Autodesk Inventor part; units mm, degrees
ref_plane "РабПлоскость6" through (0, -10.8, 0) normal (1, 0, 0) x (0, 0, -1)
ref_plane "YZ Plane" through (0, 0, 0) normal (1, 0, 0) x (0, 1, 0)
ref_plane "XZ Plane" through (0, 0, 0) normal (0, 1, 0) x (-1, 0, 0)
sketch "Эскиз1" plane through (0, 0, 0) normal (0, 0, 1) x (1, 0, 0)
  circle A0 centre (0, 0) radius 5.75
  circle A1 centre (0, 0) radius 9.55
  line L0 (9.55, 13.5) -> (-9.55, 13.5)
  line L1 (-9.55, 13.5) -> (-9.55, 0)
  line L2 (-9.55, 0) -> (9.55, 0)
  line L3 (9.55, 0) -> (9.55, 13.5)
  line L4 (9.55, 0) -> (-9.55, 0)
  line L5 (-9.55, 0) -> (-9.55, -10.8)
  line L6 (-9.55, -10.8) -> (9.55, -10.8)
  line L7 (9.55, -10.8) -> (9.55, 0)
  point P0 (9.55, 0)
  point P1 (0, 9.55)
  point P2 (-9.55, 0)
  point P3 (9.55, 0)
  point P4 (-9.55, 0)
  dimension "d0" = 11.5
  dimension "d1" = 19.1
  dimension "d64" = 10.8
  dimension "d85" = 13.5
extrude "Выдавливание1" add sketch "Эскиз1" along normal blind 8 contours L2 A1 A0 | A0 L2 A1 | L7 L6 L5 A1 | A1 L1 L0 L3
sketch "Эскиз15" plane through (0, 0, 8) normal (0, 0, 1) x (1, 0, 0)
  circle A0 centre (0, 0) radius 5.75
  circle A1 centre (0, 0) radius 7.55
  dimension "d67" = 15.1
extrude "Выдавливание9" cut sketch "Эскиз15" against normal blind 4
ref_plane "РабПлоскость6" through (0, -10.8, 0) normal (1, 0, 0) x (0, 0, -1)
sketch "Эскиз16" plane through (-9.55, -10.8, 0) normal (0, -1, 0) x (1, 0, 0)
  line L0 (0, 8) -> (19.1, 8)
  line L1 (19.1, 8) -> (24.7, 8)
  line L2 (24.7, 8) -> (24.7, 0)
  line L3 (24.7, 0) -> (19.1, 0)
  line L4 (19.1, 0) -> (19.1, 8)
  point P0 (9.55, 0)
  dimension "d70" = 5.6
  dimension "d71" = 8
extrude "Выдавливание10" add sketch "Эскиз16" against normal up to surface (24.3 mm away)
sketch "Эскиз17" plane through (-9.55, 13.5, 0) normal (0, 1, 0) x (1, 0, 0)
  line L0 (24.7, 0) -> (24.7, -8)
  line L1 (24.7, -4) -> (20.15, -4)
  point P0 (9.55, 0)
  dimension "d82" = 4.55
hole "Отверстие4" at (10.6, 13.5, 4) direction (0, -1, 0) diameter 3.2 end through all
fillet "Сопряжение5" radius 5.05 1 edges at (15.15, 1.35, 8)
fillet "Сопряжение5" radius 2.95 1 edges at (15.15, 1.35, 0)
mirror "Зеркальное отражение5" about plane through (0, -10.8, 0) normal (1, 0, 0) of "Сопряжение5", "Отверстие4", "Выдавливание10"
sketch "Эскиз18" plane through (0, 0, 8) normal (0, 0, 1) x (1, 0, 0)
  circle A0 centre (0, 0) radius 7.55
  circle A1 centre (0, 16.1) radius 7.55
  circle A2 centre (0, -16.1) radius 7.55
  dimension "d86" = 16.1
  dimension "d87" = 16.1
extrude "Выдавливание11" cut sketch "Эскиз18" against normal through all contours A1 | A2
ref_plane "РабПлоскость7" through (0, -10.8, 0) normal (1, 0, 0) x (0, 0, -1)
equation "\"d87\" = d86"
properties part number "Крепление дифференциала"
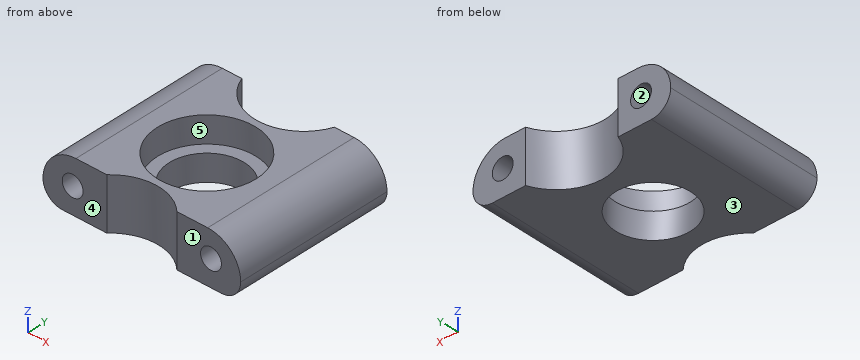
Could you check a few things on this model? Use its own coordinates, in mm. Face numbers are marked on the shaded views. A direction names the side the tool comes from. Give positions to 0.01 mm unless a question says otherwise; leave off trailing zeros. Order: outer loops, then holes, each group sorted by start corner. A loop starts at its lowest first (then second) coordinate and runs counter-clockwise, first axis right, second up.
Q1. Suppose I cut it at B-B, the plane x = 0. Write out the boundary of the cut face in (y, z).
Q2. For the marked faces 4 and 5, which set-ups out of +Z, -Z, +X, -X, +Y, -Y let a thin tool reach every point of the face, with its end or its side?
Q3. Suppose I cut it at A-A, the plane y = 0. Count the separate pieces of the cut face and the enclosed holes in it, and give its area (3 significant figures).
Q4. Suppose I cut it at C-C, the plane z = 5.25. Write out the boundary of the cut face in (x, y), and give its area (3 significant figures).
Q5. I'm going to push flat-ended pins straight in: P1, Ø1.9, axis at x = -10.6, z = 4, coming from the +Y side; P2, Ø1, axis at x = -5.5, z = 5.5, coming from the +Y side; P3, Ø1, axis at x = -1.5, z = 5.5, coming from the -Y side. Where does each tip first touch, or does it pass through?
Q6. We'd pull the mould along Z, two halves only. Please class the marked faces 1, 2 and 3: +Z half, -Z half, draft (parallel to the pull), parting line (faces both ways), or undercut.
Q7. If I drill on line 1 along X through (y, z) = (2.25, 5.25); line 2 along Y through (x, z) = (5.5, 4.5); line 3 along X through (y, z) = (12.5, 1), over which ranges is the centre line in solid material (lowest first)?
Solution:
1. outline: (-8.55, 0) - (-5.75, 0) - (-5.75, 4) - (-7.55, 4) - (-7.55, 8) - (-8.55, 8) - close; (5.75, 0) - (8.55, 0) - (8.55, 8) - (7.55, 8) - (7.55, 4) - (5.75, 4) - close
2. face 4: +Z, -Z, +X, -X, -Y
2. face 5: +Z
3. separate pieces: 2
3. enclosed holes: 2
3. area: 105 mm2
4. outline: (-14.6, -10.8) - (-11.6, -10.8) - (-11.6, 13.5) - (-14.6, 13.5) - close; (-9.6, -10.8) - (-5.38, -10.8) arc R7.55 cw to (5.38, -10.8) - (9.6, -10.8) - (9.6, 13.5) - (7.09, 13.5) arc R7.55 cw to (-7.09, 13.5) - (-9.6, 13.5) - close; (11.6, -10.8) - (14.6, -10.8) - (14.6, 13.5) - (11.6, 13.5) - close; hole circle Ø15.1 at (0, 0)
4. area: 365 mm2
5. P1: passes through
5. P2: stops at y = 11.52
5. P3: stops at y = -8.82
6. face 1: draft
6. face 2: undercut
6. face 3: -Z half
7. line 1: x = -14.6 to -11.6, -9.6 to -7.21, 7.21 to 9.6, 11.6 to 14.6
7. line 2: y = -10.8 to -5.17, 5.17 to 10.93
7. line 3: x = -14.41 to -6.64, 6.64 to 14.41
